from build123d import *

# Parameters (mm, degrees)
BOSS_EXTRUDE1_DEPTH    = 35
SKETCH4_W              = 1200
SKETCH4_H              = 806.4
BOSS_EXTRUDE2_DEPTH    = 6.35
CHAMFER1_SIZE          = 10
F_20_0MM_DOWEL_HOLE1_D = 21
CUT_EXTRUDE1_START     = -5
CUT_EXTRUDE1_DEPTH     = 5


with BuildPart() as part:
    # Sketch3 → Boss-Extrude1 (new body)
    with BuildSketch(Plane(origin=(0, 0, 0), x_dir=(1, 0, 0), z_dir=(0, 1, 0))):
        with BuildLine():
            Line((0, 531), (0, 521))
            ThreePointArc((0, 521), (-260.5, 451.199235372), (-451.199235372, 260.5))
            Line((-451.199235372, 260.5), (-459.85948941, 265.5))
            ThreePointArc((-459.85948941, 265.5), (-265.5, 459.85948941), (0, 531))
        make_face()
    extrude(amount=BOSS_EXTRUDE1_DEPTH)

    # Sketch4 → Boss-Extrude2 (add)
    with BuildSketch(Plane(origin=(0, 0, 0), x_dir=(1, 0, 0), z_dir=(0, 1, 0))):
        with Locations((-164.07, 127.8)):
            Rectangle(SKETCH4_W, SKETCH4_H)
    extrude(amount=-BOSS_EXTRUDE2_DEPTH)

    # Chamfer1
    # the kernel refuses this chamfer: 10 mm, written as the material it takes off along each edge
    with BuildSketch(Plane(origin=(0, 0, -521), x_dir=(-0.999953038196086, 0, 0.009691305506332204), z_dir=(0, 1, 0))) as chamfer1_piece_1:
        with BuildLine():
            Line((10.098340338, 0), (-CHAMFER1_SIZE * 0.00969130550632, -CHAMFER1_SIZE * 0.999953038196))
            Line((-CHAMFER1_SIZE * 0.00969130550632, -CHAMFER1_SIZE * 0.999953038196), (0, 0))
            ThreePointArc((0, 0), (5.192000536, -0.024447522), (10.098340338, 0))
        make_face()
    extrude(amount=60.969219121, mode=Mode.SUBTRACT)

    # Ø20.0mm Dowel Hole1 (through all)
    with Locations(Plane(origin=(0, 0, 0), x_dir=(1, 0, 0), z_dir=(0, 1, 0))):
        with Locations((0, 0)):
            Hole(F_20_0MM_DOWEL_HOLE1_D / 2)

    # Sketch8 → Cut-Extrude1 (cut)
    with BuildSketch(Plane(origin=(0, 0, 0), x_dir=(1, 0, 0), z_dir=(0, 1, 0)).offset(CUT_EXTRUDE1_START)):
        with BuildLine():
            Line((-462.549726308, -280.586440678), (-453.999823789, -275.4))
            ThreePointArc((-453.999823789, -275.4), (-462.708547576, 260.502975031), (0, 531))
            Line((0, 531), (0, 541))
            ThreePointArc((0, 541), (-471.422456193, 265.408869099), (-462.549726308, -280.586440678))
        make_face()
    extrude(amount=CUT_EXTRUDE1_DEPTH, mode=Mode.SUBTRACT)


solid = part.part
Here's how the part is built. I have some questions about the finished solid (model axes, mm). A direction names the side the tool comes from. Give positions to 0.01 mm unless a question says otherwise; leave off trailing zeros. Loops run counter-clockwise (first coordinate to the right, second up) from the corner with the lowest first, then second, coordinate; pieces in that order, holes last. Notation, with made-up numbers: (88.5, 35.25) -> (140.5, 35.25) arc R18 ccw to (140.5, 58.25) -> close; hole circle Ø6 at (25.5, 41). An arc over 180 degrees is marked (long way). One line per item, written item: value.
Q1. I'm going to push flat-ended pins straight in: pin 1 Ø6 at (x, z) = (162, 155) entering from +Y; pin 2 Ø17 at (x, z) = (0, 0) entering from -Y; pin 3 Ø2 at (x, y) = (-339.5, 6.5) entering from -Z. Where does each tip first touch, or does it pass through?
Answers follow:
pin 1: y = 0
pin 2: through
pin 3: z = -409.12
Q2. Suppose I cut it at B-B on x = -243.5. Please give me the cut outline in (y, z).
Answers follow:
outline: (-6.35, -531) -> (0, -531) -> (0, -483.1) -> (-5, -483.1) -> (-5, -471.88) -> (35, -471.88) -> (35, -460.6) -> (0, -460.6) -> (0, 275.4) -> (-6.35, 275.4) -> close
Q3. On a 3-axis mill with a long thin cutter (end or side, diameter ignored), from which of +Z, -Z, +X, -X, +Y, -Y can I reach the whole of each face in a straight line? I mean faces 1 (the face through (-472, -5, -249)), 2 (the face through (-172, -6.35, -133)), 3 (the face through (-54, 0, -133)). Say none if no direction works.
Answers follow:
face 1: +Y
face 2: +Z, -Z, +X, -X, -Y
face 3: +Z, +X, +Y
Q4. If I drill on line 1 along Z through (x, y) = (0, -2); line 2 along Y through (x, z) = (-285.5, -98); line 3 along X through (y, z) = (-3, 216), over which ranges is the centre line in solid material (lowest first)?
Answers follow:
line 1: -531 to -10.5, 10.5 to 275.4
line 2: -6.35 to 0
line 3: -764.07 to -496.01, -485.08 to 435.93
Q5. Suppose I cut it at D-D on z = -54. Please give me the cut outline in (x, y), then the cut area to 3 significant figures.
Answers follow:
outline: (-764.07, -6.35) -> (435.93, -6.35) -> (435.93, 0) -> (-528.25, 0) -> (-528.25, -5) -> (-538.3, -5) -> (-538.3, 0) -> (-764.07, 0) -> close
area: 7,570 mm^2
Q6. Suppose I cut it at C-C on y = 22.5. Please give me the cut outline in (x, z).
Answers follow:
outline: (-459.86, -265.5) arc R531 ccw to (0, -531) -> (-10.1, -520.9) arc R521 cw to (-451.2, -260.5) -> close
Q7. We'd pull the mould along Z, two halves only. Please class faces 4 (the face through (-490.51, -2.54, -228.21)), 5 (the face through (-261.626, 17.255, -450.547)), 6 (the face through (-585, 0, -223)): pulls with the +Z half, pulls with the -Z half, needs draft (parallel to the pull), parting line crosses it, or undercut.
Answers follow:
face 4: undercut
face 5: pulls with the +Z half
face 6: needs draft
Q8. Suppose I cut it at A-A on z = -151. Please give me the cut outline in (x, y).
Answers follow:
outline: (-764.07, -6.35) -> (435.93, -6.35) -> (435.93, 0) -> (-509.08, 0) -> (-509.08, -5) -> (-519.5, -5) -> (-519.5, 0) -> (-764.07, 0) -> close
